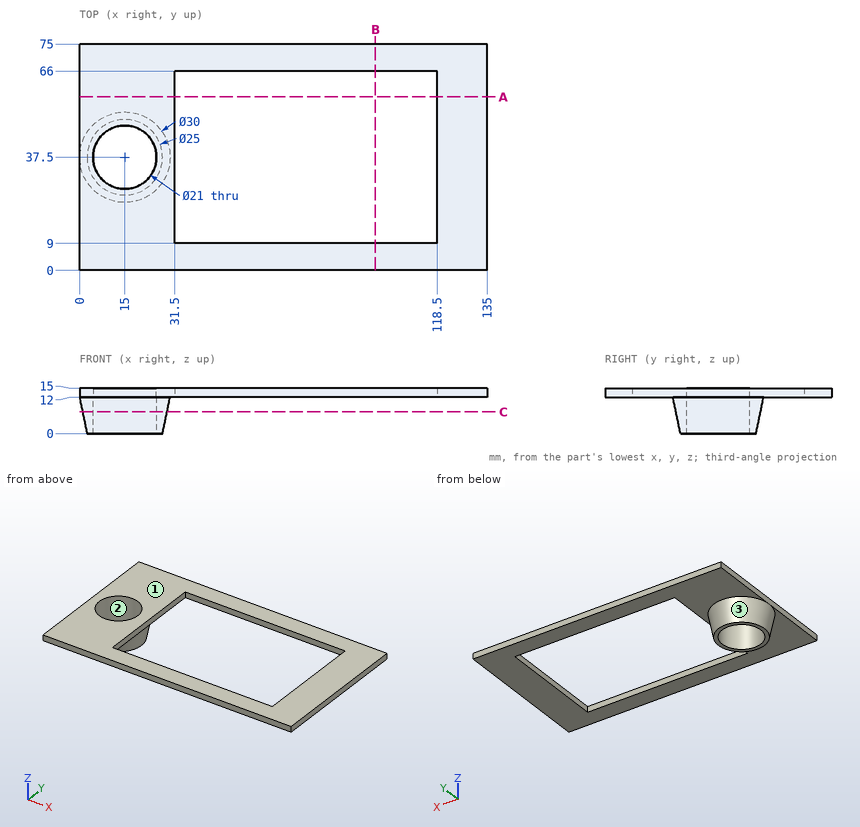
Print and shaded views of the part. All mm, measured from the part's lowest x, y and z. Round coordinates to 2 decimals unless told otherwise and drop trailing zeros. Write each loop counter-clockwise with the first axis right and the second up, starting at its lowest first coordinate (ties: lowest second). Pieces come first, ordered by that corner, then holes. Notation, with made-up numbers: (24, -13) -> (46, -13) arc R16 cw to (46, 15) -> close; hole circle Ø6 at (64.25, -3.75). An arc over 180 degrees is marked (long way). Write item = value, one per line.
(1) Band-saw the part on B-B (x = 98). Give the cut face in (y, z), then the cut area to 3 significant figures.
Answer:
outline = (0, 12) -> (9, 12) -> (9, 15) -> (0, 15) -> close; (66, 12) -> (75, 12) -> (75, 15) -> (66, 15) -> close
area = 54.0 mm2
(2) Probe L1, parallel to X at y = 24.5, z = 12.75; L2, parallel to Y at x = 52, z = 13.5; L3, parallel to Z at x = 23, y = 20. List the from-to ranges inside material, lowest first.
Answer:
L1 = 0 to 31.5, 118.5 to 135
L2 = 0 to 9, 66 to 75
L3 = 12 to 15
(3) Flat gauge pin, fed straight in: pin 1 (4 mm diameter, centred on y = 29, z = 8.5, fed in from -X). Where does the tip first touch, or does it go through?
Answer:
pin_1 = 2.19
(4) Band-saw the part on C-C (z = 7.25). Give the cut face in (x, y), then the cut area to 3 significant figures.
Answer:
outline = circle Ø28.02 at (15, 37.5); hole circle Ø21 at (15, 37.5)
area = 270 mm2
(5) Two-plate mould, pull along X, no slides. Class the marked faces 1, 2 and 3: pulls with the +X half, pulls with the -X half, needs draft (parallel to the pull), parting line crosses it, or undercut.
Answer:
face_1 = needs draft
face_2 = undercut
face_3 = parting line crosses it
(6) Band-saw the part on A-A (y = 57.5). Give the cut face in (x, z), then the cut area to 3 significant figures.
Answer:
outline = (0, 12) -> (31.5, 12) -> (31.5, 15) -> (0, 15) -> close; (118.5, 12) -> (135, 12) -> (135, 15) -> (118.5, 15) -> close
area = 144 mm2
